Can you work these out from the model? Positions are in its coordinate system, mm. A direction names the side the tool comes from. Give positions to 0.01 mm unless a question says otherwise; leave off trailing zeros. Order: outer loops, then holes, each group sorted by start corner. A loop starts at its lowest first (then second) coordinate and runs counter-clockwise, first axis right, second up. Notation, with made-up numbers: (78.5, -20) - (92.5, -20) arc R19 cw to (92.5, 12) - close; hole circle Ø6 at (88, 36.5). An arc over 180 degrees is marked (long way). One line per question, with ' | ' between items.
```python
from build123d import *

# Parameters (mm, degrees)
SKETCH1_R           = 9
SKETCH1_R_2         = 7
BOSS_EXTRUDE1_DEPTH = 12
BOSS_EXTRUDE2_START = -0.937742
SKETCH2_W           = 8
SKETCH2_H           = 12
BOSS_EXTRUDE2_DEPTH = 1.437742
BOSS_EXTRUDE3_DEPTH = 8
SKETCH4_R           = 2
CUT_EXTRUDE1_DEPTH  = 11
CIRPATTERN1_COUNT   = 3
FILLET1_R           = 2
FILLET2_R           = 0.5


with BuildPart() as part:
    # Sketch1 → Boss-Extrude1 (new body)
    with BuildSketch(Plane(origin=(0, 0, 0), x_dir=(1, 0, 0), z_dir=(0, 1, 0))):
        with Locations(Location((0, 0, 0), (0, 0, 270))):
            Circle(SKETCH1_R)
        with Locations(Location((0, 0, 0), (0, 0, 270))):
            Circle(SKETCH1_R_2, mode=Mode.SUBTRACT)
    extrude(amount=BOSS_EXTRUDE1_DEPTH)

    # Sketch2 → Boss-Extrude2 (add)
    with BuildSketch(Plane.XY.offset(9).offset(BOSS_EXTRUDE2_START)):
        with Locations((0, 6)):
            Rectangle(SKETCH2_W, SKETCH2_H)
    boss_extrude2 = extrude(amount=BOSS_EXTRUDE2_DEPTH)

    # Sketch3 → Boss-Extrude3 (add)
    with BuildSketch(Plane.ZY.offset(4)):
        Polygon((9.5, 0), (12.5, 0), (15.5, 0), (15.5, 12), (14, 12), (14, 3), (11, 3), (11, 12), (9.5, 12), align=None)
    boss_extrude3 = extrude(amount=-BOSS_EXTRUDE3_DEPTH)

    # Sketch4 → Cut-Extrude1 (cut)
    with BuildSketch(Plane.ZY.offset(4)):
        with Locations((12.5, 3)):
            Circle(SKETCH4_R)
    cut_extrude1 = extrude(amount=-CUT_EXTRUDE1_DEPTH, mode=Mode.SUBTRACT)

    # CirPattern1: Boss-Extrude2, Boss-Extrude3, Cut-Extrude1 ×3 about axis
    cirpattern1_axis = Axis((0, 0, 0), (0, 1, 0))
    add([boss_extrude2.rotate(cirpattern1_axis, i * 360 / CIRPATTERN1_COUNT) for i in range(1, CIRPATTERN1_COUNT)])
    add([boss_extrude3.rotate(cirpattern1_axis, i * 360 / CIRPATTERN1_COUNT) for i in range(1, CIRPATTERN1_COUNT)])
    add([cut_extrude1.rotate(cirpattern1_axis, i * 360 / CIRPATTERN1_COUNT) for i in range(1, CIRPATTERN1_COUNT)], mode=Mode.SUBTRACT)

    # Fillet1
    fillet1_edges = [part.edges().sort_by_distance(p)[0] for p in [
        (-13.423393759, 0, -7.75),
        (4, 6, 8.062258),
        (-4, 6, 8.062258),
        (0, 0, 15.5),
        (4.98212024, 6, -7.495230615),
        (-4.98212024, 6, -7.495230615),
        (13.423393759, 0, -7.75),
    ]]
    fillet(fillet1_edges, radius=FILLET1_R)

    # Fillet2
    fillet2_edges = [part.edges().sort_by_distance(p)[0] for p in [
        (-12.124355653, 12, -7),
        (0, 12, 11),
        (0, 12, 14),
        (9.526279442, 12, -5.5),
        (12.124355653, 12, -7),
        (-9.526279442, 12, -5.5),
    ]]
    fillet(fillet2_edges, radius=FILLET2_R)


solid = part.part
```
(1) Will these pins go through, and if not, where does the flat tip stop? pin 1 (1 mm diameter, centred on x = -10.5, y = 4, fed in from +Z); pin 2 (2 mm diameter, centred on x = -4, y = 9, fed in from -Z); pin 3 (6.5 mm diameter, centred on y = 3, z = 12.5, fed in from +X).
Answer below:
pin 1: z = -1.15 | pin 2: z = -8.49 | pin 3: x = 4
(2) If we mould it in two halves opening along Z, with no side actions, what happens to faces 1 (the face through (-11, 1, -6)), 2 (the face through (0, 6, -9)), 3 (the face through (13, 12, -7))? For each: released by +Z, released by -Z, zero draft, split by the parting line, or undercut.
Answer below:
face 1: undercut | face 2: released by -Z | face 3: zero draft
(3) If I drill on line 1 (X direction, y = 8.25, z = 0); line 2 (X direction, y = 8.5, z = -7.5); line 3 (Z direction, x = 1.5, y = 8), over which ranges is the centre line in solid material (lowest first)?
Answer below:
line 1: -9 to -7, 7 to 9 | line 2: -13.57 to -11.84, -8.37 to 8.37, 11.84 to 13.57 | line 3: -8.87 to -6.84, 6.84 to 11, 14 to 15.5
(4) Imagine slicing it at D-D (z = 12.5). List the corners of the cut face in (x, y) for me.
Answer below:
outline: (-4, 0) - (4, 0) - (4, 1) - (-4, 1) - close
(5) On a 3-axis mill with a long thin cutter (end or side, diameter ignored), from which of +Z, -Z, +X, -X, +Y, -Y can I reach the whole of each face in a straight line? I mean faces 4 (the face through (-4.25, 6.08, 8.25)), 5 (the face through (9.554, 7.861, -5.452)), 6 (the face through (0, 8, 14)), 7 (the face through (4, 6, 10)). Say none if no direction works.
Answer below:
face 4: +Z, -X, +Y, -Y | face 5: +Y | face 6: +X, -X, +Y | face 7: +Z, +X, +Y, -Y
(6) Imagine slicing it at A-A (y = 10.5). Count the separate pieces of the cut face and the enclosed holes in it, and give its area (3 significant figures).
Answer below:
separate pieces: 4 | enclosed holes: 1 | area: 193 mm^2
(7) Imagine slicing it at B-B (z = 0). List the corners of the cut face in (x, y) for me, and give its area (3 significant figures).
Answer below:
outline: (-9, 0) - (-7, 0) - (-7, 12) - (-9, 12) - close; (7, 0) - (9, 0) - (9, 12) - (7, 12) - close | area: 48.0 mm^2
